Design review of the part built by this model. Coordinates are the model's own, in mm. Give positions to 0.01 mm unless a question says otherwise; leave off trailing zeros. Loops run counter-clockwise (first coordinate to the right, second up) from the corner with the lowest first, then second, coordinate; pieces in that order, holes last. Notation, with made-up numbers: (-37, 43.5) -> (16, 43.5) arc R26 ccw to (16, 80.5) -> close; hole circle Ø3 at (46, 31). An arc over 180 degrees is marked (long way). Use a Markdown table: item, result. Add a question column.
1. Add section D-D (z = 1). Count the separate pieces of the cut face and the enclosed holes in it, and give its area (3 significant figures).
2. Add section C-C (y = 8). State the section outline as (x, z) points, and give its area (3 significant figures).
3. Add section B-B (x = -10). State the section outline as (y, z) points (3 decimals), and give its area (3 significant figures).
4. Add section A-A (y = 23.5). State the section outline as (x, z) points.
5. To check wall thickness, follow line 1 (Y direction, x = -23.5, z = 1.85) (3 decimals); line 2 (X direction, y = -26, z = 1.55); line 3 (X direction, y = -37, z = 0.1). State the ranges of each line that lie inside material, in increasing order.
```python
from build123d import *

# Parameters (mm, degrees)
IZIM1_W                     = 92.4
IZIM1_H                     = 94.45
IZIM1_W_2                   = 20.6
IZIM1_H_2                   = 10.45
IZIM1_W_3                   = 43.2
IZIM1_H_3                   = 10
IZIM1_H_4                   = 15
Y_KSEKLIK_EKSTR_ZYON1_DEPTH = 2
RADYUS1_R                   = 2


with BuildPart() as part:
    # Çizim1 → Yükseklik-Ekstrüzyon1 (new body)
    with BuildSketch(Plane.XY):
        Rectangle(IZIM1_W, IZIM1_H)
        with Locations((-33.9, 40)):
            Rectangle(IZIM1_W_2, IZIM1_H_2, mode=Mode.SUBTRACT)
        with Locations((-22.6, -40.225)):
            Rectangle(IZIM1_W_3, IZIM1_H_3, mode=Mode.SUBTRACT)
        with Locations((22.6, -40.225)):
            Rectangle(IZIM1_W_3, IZIM1_H_3, mode=Mode.SUBTRACT)
        with Locations((-33.9, -25.725)):
            Rectangle(IZIM1_W_2, IZIM1_H_4, mode=Mode.SUBTRACT)
        with Locations((-22.6, -8.725)):
            Rectangle(IZIM1_W_3, IZIM1_H_4, mode=Mode.SUBTRACT)
        with Locations((-33.9, 8.275)):
            Rectangle(IZIM1_W_2, IZIM1_H_4, mode=Mode.SUBTRACT)
        with Locations((-22.6, 25.275)):
            Rectangle(IZIM1_W_3, IZIM1_H_4, mode=Mode.SUBTRACT)
        with Locations((33.9, -25.725)):
            Rectangle(IZIM1_W_2, IZIM1_H_4, mode=Mode.SUBTRACT)
        with Locations((22.6, -8.725)):
            Rectangle(IZIM1_W_3, IZIM1_H_4, mode=Mode.SUBTRACT)
        with Locations((33.9, 8.275)):
            Rectangle(IZIM1_W_2, IZIM1_H_4, mode=Mode.SUBTRACT)
        with Locations((22.6, 25.275)):
            Rectangle(IZIM1_W_3, IZIM1_H_4, mode=Mode.SUBTRACT)
        with Locations((33.9, 40)):
            Rectangle(IZIM1_W_2, IZIM1_H_2, mode=Mode.SUBTRACT)
        with Locations((0, 40)):
            Rectangle(IZIM1_W_3, IZIM1_H_2, mode=Mode.SUBTRACT)
        with Locations((0, 8.275)):
            Rectangle(IZIM1_W_3, IZIM1_H_4, mode=Mode.SUBTRACT)
        with Locations((0, -25.725)):
            Rectangle(IZIM1_W_3, IZIM1_H_4, mode=Mode.SUBTRACT)
    extrude(amount=Y_KSEKLIK_EKSTR_ZYON1_DEPTH)

    # Radyus1
    radyus1_edges = [part.edges().sort_by_distance(p)[0] for p in [
        (1, -16.225, 1),
        (44.2, -16.225, 1),
        (44.2, -1.225, 1),
        (1, -1.225, 1),
        (-44.2, 15.775, 1),
        (-44.2, 0.775, 1),
        (-23.6, 0.775, 1),
        (-23.6, 15.775, 1),
        (23.6, 0.775, 1),
        (44.2, 0.775, 1),
        (44.2, 15.775, 1),
        (23.6, 15.775, 1),
        (-44.2, 32.775, 1),
        (-44.2, 17.775, 1),
        (-1, 17.775, 1),
        (-1, 32.775, 1),
        (44.2, 45.225, 1),
        (1, 17.775, 1),
        (44.2, 17.775, 1),
        (44.2, 32.775, 1),
        (1, 32.775, 1),
        (23.6, 45.225, 1),
        (23.6, 34.775, 1),
        (44.2, 34.775, 1),
        (-21.6, 34.775, 1),
        (21.6, 34.775, 1),
        (21.6, 45.225, 1),
        (-21.6, 45.225, 1),
        (-21.6, 0.775, 1),
        (21.6, 0.775, 1),
        (21.6, 15.775, 1),
        (-21.6, 15.775, 1),
        (21.6, -18.225, 1),
        (-21.6, -18.225, 1),
        (-21.6, -33.225, 1),
        (21.6, -33.225, 1),
        (-44.2, -35.225, 1),
        (-44.2, -45.225, 1),
        (-1, -45.225, 1),
        (-1, -35.225, 1),
        (-23.6, 45.225, 1),
        (-44.2, 45.225, 1),
        (-44.2, 34.775, 1),
        (-23.6, 34.775, 1),
        (1, -45.225, 1),
        (44.2, -45.225, 1),
        (44.2, -35.225, 1),
        (1, -35.225, 1),
        (-44.2, -18.225, 1),
        (-44.2, -33.225, 1),
        (-23.6, -33.225, 1),
        (-23.6, -18.225, 1),
        (46.2, -47.225, 1),
        (-46.2, -47.225, 1),
        (23.6, -33.225, 1),
        (-46.2, 47.225, 1),
        (44.2, -33.225, 1),
        (44.2, -18.225, 1),
        (23.6, -18.225, 1),
        (46.2, 47.225, 1),
        (-44.2, -1.225, 1),
        (-44.2, -16.225, 1),
        (-1, -16.225, 1),
        (-1, -1.225, 1),
    ]]
    fillet(radyus1_edges, radius=RADYUS1_R)


solid = part.part
```
Taken from the geometry:
| question | item | result |
|---|---|---|
| 1 | separate pieces | 1 |
| 1 | enclosed holes | 15 |
| 1 | area | 1,910 mm^2 |
| 2 | outline | (-46.2, 0) -> (-44.2, 0) -> (-44.2, 2) -> (-46.2, 2) -> close; (-23.6, 0) -> (-21.6, 0) -> (-21.6, 2) -> (-23.6, 2) -> close; (21.6, 0) -> (23.6, 0) -> (23.6, 2) -> (21.6, 2) -> close; (44.2, 0) -> (46.2, 0) -> (46.2, 2) -> (44.2, 2) -> close |
| 2 | area | 16.0 mm^2 |
| 3 | outline | (-47.225, 0) -> (-45.225, 0) -> (-45.225, 2) -> (-47.225, 2) -> close; (-35.225, 0) -> (-33.225, 0) -> (-33.225, 2) -> (-35.225, 2) -> close; (-18.225, 0) -> (-16.225, 0) -> (-16.225, 2) -> (-18.225, 2) -> close; (-1.225, 0) -> (0.775, 0) -> (0.775, 2) -> (-1.225, 2) -> close; (15.775, 0) -> (17.775, 0) -> (17.775, 2) -> (15.775, 2) -> close; (32.775, 0) -> (34.775, 0) -> (34.775, 2) -> (32.775, 2) -> close; (45.225, 0) -> (47.225, 0) -> (47.225, 2) -> (45.225, 2) -> close |
| 3 | area | 28.0 mm^2 |
| 4 | outline | (-46.2, 0) -> (-44.2, 0) -> (-44.2, 2) -> (-46.2, 2) -> close; (-1, 0) -> (1, 0) -> (1, 2) -> (-1, 2) -> close; (44.2, 0) -> (46.2, 0) -> (46.2, 2) -> (44.2, 2) -> close |
| 5 | line 1 | y = -47.225 to -45.225, -35.225 to -16.225, -1.225 to 17.775, 32.775 to 47.225 |
| 5 | line 2 | x = -46.2 to -44.2, -23.6 to -21.6, 21.6 to 23.6, 44.2 to 46.2 |
| 5 | line 3 | x = -46.2 to -44.19, -1.01 to 1.01, 44.19 to 46.2 |
